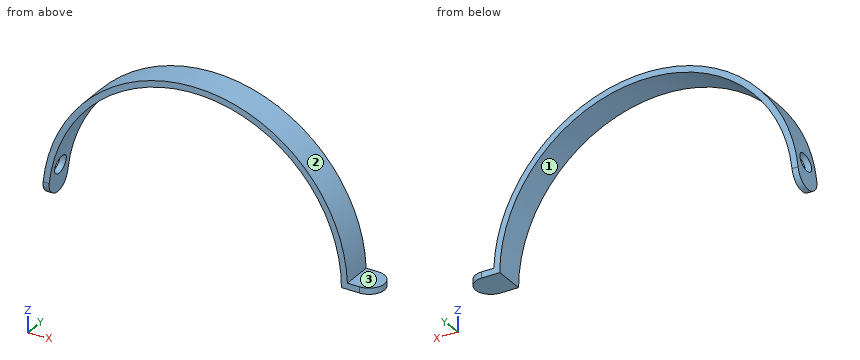
Autodesk Inventor part; units mm, degrees
ref_plane "Work Plane1" through (-25, 0, 0) normal (1, 0, 0) x (0, 1, 0)
ref_plane "XZ Plane" through (0, 0, 0) normal (0, 1, 0) x (-1, 0, 0)
ref_plane "XY Plane" through (0, 0, 0) normal (0, 0, 1) x (1, 0, 0)
sketch "Sketch1" plane through (0, 0, 0) normal (0, 1, 0) x (-1, 0, 0)
  arc A0 (25, 0) -> (-24.98, 1) centre (0, 0) ccw
  arc A1 (24, 0) -> (-24, 0) centre (0, 0) ccw
  line L0 (25, 0) -> (24, 0)
  line L1 (-24, 0) -> (-25, 0)
  line L2 (-24, 0) -> (-29.5, 0)
  line L3 (-29.5, 0) -> (-29.5, 1)
  line L4 (-29.5, 1) -> (-24.98, 1)
  line L5 (-24, 1) -> (-24, 0)
extrude "Extrusion1" add sketch "Sketch1" along normal blind 5
sketch "Sketch2" plane through (29.5, 0, 0) normal (0, 0, -1) x (-1, 0, 0)
  line L0 (0, 0) -> (5.5, 0)
  arc A0 (2.5, 5) -> (2.5, 0) centre (2.5, 2.5) ccw
  line L1 (0, 0) -> (2.5, 0)
  line L2 (4.52, 0) -> (0, 0)
  line L3 (0, 0) -> (0, 2.5)
  line L4 (0, 0) -> (0, 5)
  line L5 (0, 2.5) -> (0, 5)
  line L6 (0, 5) -> (2.26, 5)
  line L7 (4.52, 5) -> (0, 5)
  line L8 (2.5, 5) -> (0, 5)
  line L9 (0, 2.5) -> (0, 5)
  line L10 (0, 2.5) -> (0, 0)
  line L11 (0, 0) -> (2.5, 0)
  arc A1 (0, 2.5) -> (2.5, 0) centre (2.5, 2.5) ccw
  arc A2 (2.5, 5) -> (0, 2.5) centre (2.5, 2.5) ccw
  point P0 (29.5, 0)
extrude "Extrusion2" cut sketch "Sketch2" against normal through all
ref_plane "Work Plane1" through (-25, 0, 0) normal (1, 0, 0) x (0, 1, 0)
sketch "Sketch3" plane through (-25, 0, 0) normal (1, 0, 0) x (0, 1, 0)
  line L0 (5, 0) -> (5, 25) construction
  line L1 (0, 0) -> (0, 2) construction
  line L2 (0, 0) -> (0, 25) construction
  line L3 (0, 0) -> (0, 2.5) construction
  arc A0 (0, 2.5) -> (5, 2.5) centre (2.5, 2.5) ccw
  line L4 (0, 0) -> (0, 2.5)
  line L5 (0, 0) -> (5, 0)
  line L6 (0, 0) -> (2.5, 0)
  line L7 (2.5, 0) -> (5, 0)
  line L8 (5, 0) -> (5, 2.5)
  arc A1 (0, 2.5) -> (2.5, 0) centre (2.5, 2.5) ccw
  arc A2 (2.5, 0) -> (5, 2.5) centre (2.5, 2.5) ccw
  point P0 (0, 1)
  point P1 (5, 1)
extrude "Extrusion3" cut sketch "Sketch3" along normal blind 3
sketch "Sketch4" plane through (-25, 0, 0) normal (1, 0, 0) x (0, 1, 0)
  line L0 (0, 0) -> (0, 4.5) construction
  line L1 (0, 24) -> (0, 0) construction
  line L2 (0, 4.5) -> (5, 4.5) construction
  line L3 (5, 24) -> (5, 0) construction
  circle A0 centre (2.5, 4.5) radius 1.5
  point P0 (0, 2.5)
  point P1 (5, 2.5)
  dimension "d15" = 4.5
  dimension "d16" = 3
extrude "Extrusion4" cut sketch "Sketch4" along normal blind 4
properties part number "Metal icecream cutter"
Geometry check sheet. Reference: the model listing, model coordinates, mm. Face numbers are marked on the shaded views. Round coordinates to 2 decimals unless told otherwise and drop trailing zeros. Order: outer loops, then holes, each group sorted by start corner. A loop starts at its lowest first (then second) coordinate and runs counter-clockwise, first axis right, second up. Notation, with made-up numbers: M 70.25,-16 L 75.25,-16 A16 cw 75.25,-5 Z; hole C 37,-31 d8. An arc over 180 degrees is marked long. Answer in a Markdown table with one row per item. Add a question column.
Item 1: Material ranges on L1, parallel to Y at x = -23.8, z = 4.5; L2, parallel to X at y = 1.1, z = 14; L3, parallel to X at y = 0.75, z = 6, recorded low to high. Write a range as [from, to].
Item 2: Sectioned sample at D-D, the plane z = 19.75. Enter the section's corners in (x, y), plus the area to 3 significant figures.
Item 3: Depth check by flat-ended pin: pin 1 Ø1 at (x, y) = (14, 0.5) entering from -Z; pin 2 Ø1.5 at (x, y) = (-14.5, 4) entering from -Z; pin 3 Ø2.5 at (x, y) = (28, 3.5) entering from +Z. Enter the tip coordinate at first touch or a pass-through.
Item 4: Draft check along X on the marked faces 1, 2 and 3. Enter one of: released by +X, released by -X, zero draft, split by the parting line, or undercut.
Item 5: Sectioned sample at C-C, the plane z = 4.5. Enter the section's corners in (x, y), plus the area to 3 significant figures.
Item 6: Sectioned sample at B-B, the plane y = 2.5. Enter the section's corners in (x, z), plus the area to 3 significant figures.
Item 7: Sectioned sample at A-A, the plane z = 15.75. Enter the section's corners in (x, y).
Filled in:
| question | item | result |
|---|---|---|
| 1 | L1 | y = [0, 1], [4, 5] |
| 1 | L2 | x = [-20.71, -19.49], [19.49, 20.71] |
| 1 | L3 | x = [-24.27, -23.24], [23.24, 24.27] |
| 2 | outline | M -15.33,0 L -13.64,0 L -13.64,5 L -15.33,5 Z; M 13.64,0 L 15.33,0 L 15.33,5 L 13.64,5 Z |
| 2 | area | 16.9 mm² |
| 3 | pin 1 | stops at z = 19.12 |
| 3 | pin 2 | stops at z = 18.53 |
| 3 | pin 3 | stops at z = 1 |
| 4 | face 1 | undercut |
| 4 | face 2 | split by the parting line |
| 4 | face 3 | zero draft |
| 5 | outline | M -24.59,0 L -23.57,0 L -23.57,1 L -24.59,1 Z; M -24.59,4 L -23.57,4 L -23.57,5 L -24.59,5 Z; M 23.57,0 L 24.59,0 L 24.59,5 L 23.57,5 Z |
| 5 | area | 7.12 mm² |
| 6 | outline | M -25,0 L -24,0 A24 cw -23.81,3 L -24.82,3 A25 ccw Z; M -24.27,6 L -23.24,6 A24 cw 24,0 L 29.5,0 L 29.5,1 L 24.98,1 A25 ccw Z |
| 6 | area | 78.4 mm² |
| 7 | outline | M -19.41,0 L -18.11,0 L -18.11,5 L -19.41,5 Z; M 18.11,0 L 19.41,0 L 19.41,5 L 18.11,5 Z |
